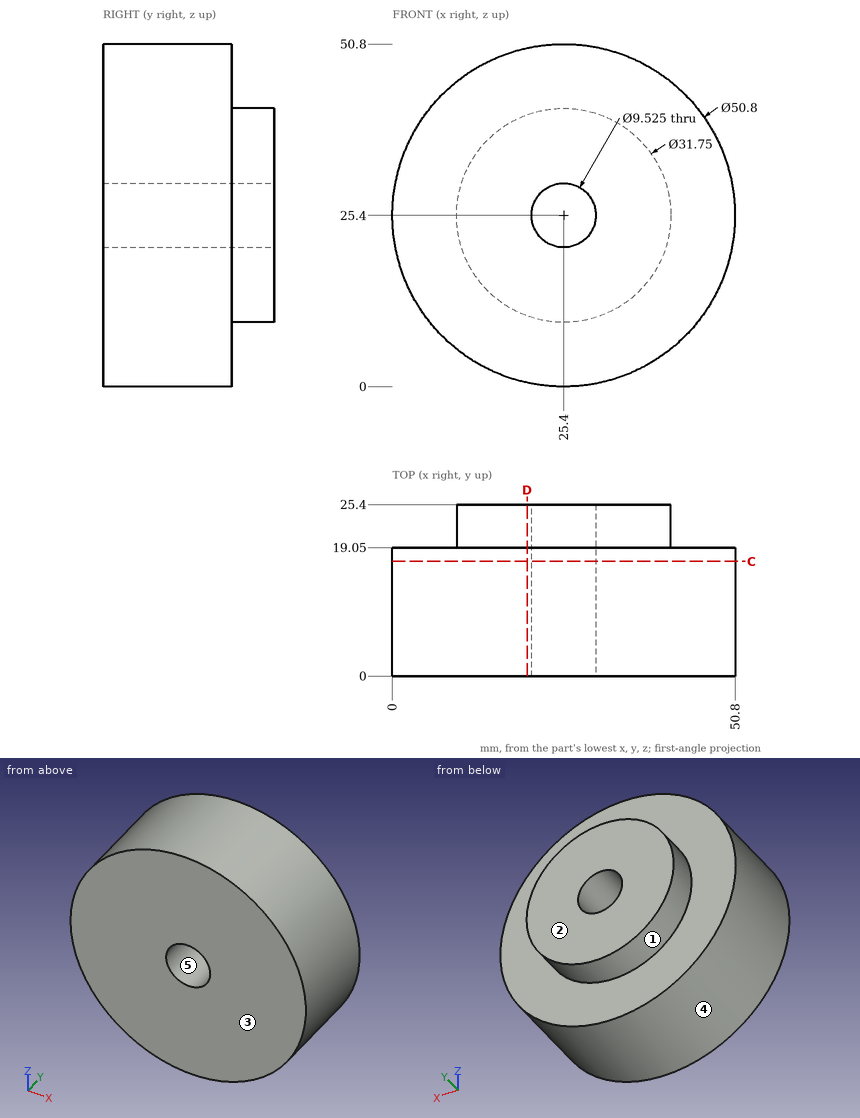
The drawing under review shows one solid part. Ordinate dimensions are in mm from its lowest x, y, z. A direction names the side the tool comes from. Round coordinates to 2 decimals unless told otherwise and drop trailing zeros. Loops run counter-clockwise (first coordinate to the right, second up) from the corner with the lowest first, then second, coordinate; pieces in that order, holes last.
Item 1: For the marked faces 1 and 2, list the 3-axis set-ups (+Z, -Z, +X, -X, +Y, -Y) from which the entire face can be reached by the end or side of a thin tool; tool diameter is ignored.
Determined:
face 1: +Y
face 2: +Z, -Z, +X, -X, +Y
Item 2: Clearance check with flat-ended pins moving along their axes: pin 1 Ø4 at (x, z) = (32.5, 36.5) entering from -Y; pin 2 Ø2 at (x, y) = (31, 21.5) entering from +Z; pin 3 Ø8 at (x, y) = (29, 16) entering from +Z; pin 4 Ø4 at (x, y) = (35.5, 15) entering from -Z. State where each tip first meets the part, or that it passes through.
Determined:
pin 1: stops at y = 0
pin 2: stops at z = 40.59
pin 3: stops at z = 50.8
pin 4: stops at z = 1.33
Item 3: Take a section at C-C (y = 17). Write out the cut boundary in (x, z) (1 decimal).
Determined:
outline: circle Ø50.8 at (25.4, 25.4); hole circle Ø9.5 at (25.4, 25.4)
Item 4: For line 1 (Z direction, x = 25.4, y = 15.5); line 2 (Y direction, x = 18, z = 7); line 3 (Z direction, x = 24.5, y = 11.25), list the stretches that pass through material, from the lowest coordinate up.
Determined:
line 1: z = 0 to 20.64, 30.16 to 50.8
line 2: y = 0 to 19.05
line 3: z = 0.02 to 20.72, 30.08 to 50.78
Item 5: Take a section at D-D (x = 20). Write out the cut boundary in (y, z).
Determined:
outline: (0, 0.58) - (19.05, 0.58) - (19.05, 10.47) - (25.4, 10.47) - (25.4, 40.33) - (19.05, 40.33) - (19.05, 50.22) - (0, 50.22) - close
Item 6: Mouldability with a two-part tool opening along Z and no side actions: class the marked faces 3, 4 and 5 as released by +Z, released by -Z, zero draft, split by the parting line, or undercut.
Determined:
face 3: zero draft
face 4: split by the parting line
face 5: undercut
